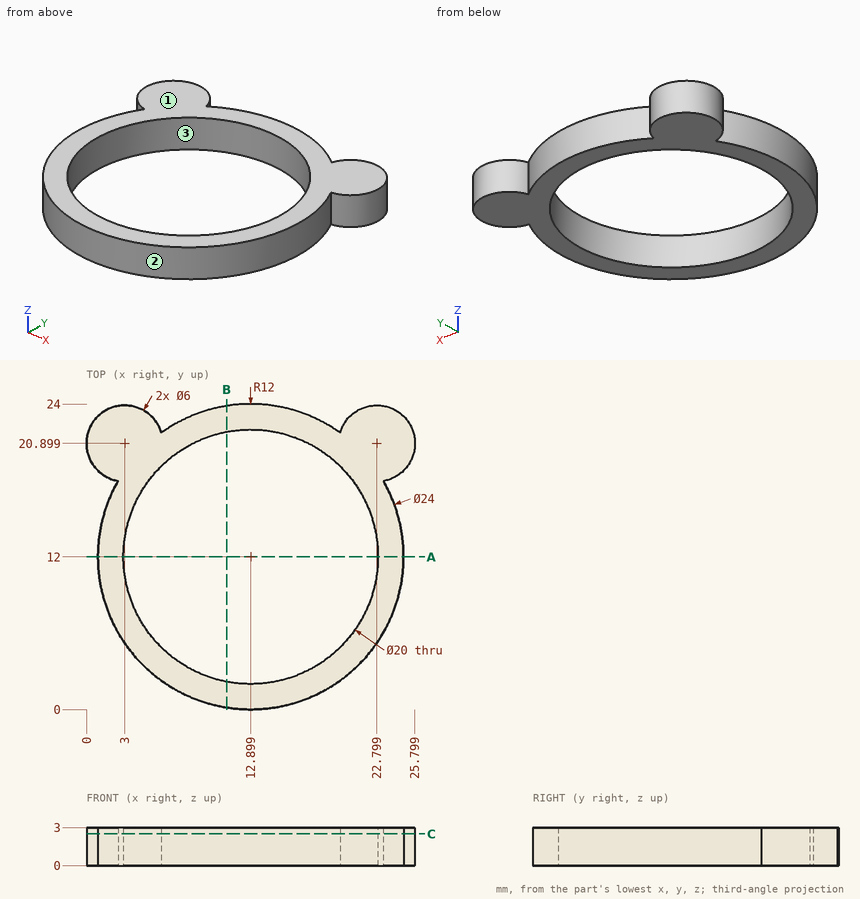
Check sheet for the drawn part. Datum: minimum x, y, z corner. Units: mm. Round coordinates to 2 decimals unless told otherwise and drop trailing zeros. Loops run counter-clockwise (first coordinate to the right, second up) from the corner with the lowest first, then second, coordinate; pieces in that order, holes last. Notation, with made-up numbers: (66, -38) - (105, -38) arc R21 cw to (105, 0) - close; hole circle Ø3 at (87.25, 53). An arc over 180 degrees is marked (long way). Write each question's results on one line, items separated by ' | '. Start each with the question number.
Q1. Gauge pin test, flat end, axial feed: P1, Ø8, axis at x = 11.5, y = 10.5, coming from the +Z side. Record the tip position at first contact, or that the pin passes through.
Q2. Cross-section at A-A on y = 12. Enter the section's corners in (x, z), and give its area (3 significant figures).
Q3. Cross-section at B-B on x = 11. Enter the section's corners in (y, z).
Q4. Cross-section at C-C on z = 2.5. Enter the section's corners in (x, y) (1 decimal), and give its area (3 significant figures).
Q5. Release check for a two-part mould opening along Y. For the marked faces 1, 2 and 3 record: +Y half, -Y half, draft (parallel to the pull), parting line (faces both ways), or undercut.
Q6. Thickness scan on line 1 (X direction, y = 12, z = 1.65); line 2 (Y direction, x = 12.75, z = 2.05); line 3 (X direction, y = 11, z = 1.4). Record the ranges inside material, lowest first. Write a range as [from, to].
Answers below:
1) P1: passes through
2) outline: (0.9, 0) - (2.9, 0) - (2.9, 3) - (0.9, 3) - close; (22.9, 0) - (24.9, 0) - (24.9, 3) - (22.9, 3) - close | area: 12.0 mm²
3) outline: (0.15, 0) - (2.18, 0) - (2.18, 3) - (0.15, 3) - close; (21.82, 0) - (23.85, 0) - (23.85, 3) - (21.82, 3) - close
4) outline: (2.5, 17.9) arc R12 ccw (long way) to (23.3, 17.9) arc R3 ccw (long way) to (19.9, 21.7) arc R12 ccw to (5.9, 21.7) arc R3 ccw (long way) to start; hole circle Ø20 at (12.9, 12) | area: 183 mm²
5) face 1: draft | face 2: undercut | face 3: undercut
6) line 1: x = [0.9, 2.9], [22.9, 24.9] | line 2: y = [0, 2], [22, 24] | line 3: x = [0.94, 2.95], [22.85, 24.86]
